Work out the finished part from the listing and answer in its coordinate system (mm). A direction names the side the tool comes from. Coordinates: 2 decimals unless noted, no trailing zeros. Loops run counter-clockwise (first coordinate to the right, second up) from the corner with the lowest first, then second, coordinate; pieces in that order, holes last. Notation, with made-up numbers: (21.25, 40.25) -> (69.25, 40.25) arc R16 cw to (69.25, 57.25) -> close; hole circle Ø3 at (-1, -10). An arc over 180 degrees is marked (long way). Use a Markdown table: item, result. Add a question column.
```python
from build123d import *

# Parameters (mm, degrees)
SKETCH8_W               = 3.38
SKETCH8_H               = 38.1
BOSS_EXTRUDE10_DEPTH    = 43.18
CUT_EXTRUDE7_DEPTH      = 71.315115907
CUT_EXTRUDE7_DEPTH_BACK = 71.315115907
SKETCH18_R              = 3.175
SKETCH23_R              = 3.175
CUT_EXTRUDE9_DEPTH      = 71.315115907


with BuildPart() as part:
    # Sketch2 → Revolve1 (revolve)
    with BuildSketch(Plane(origin=(0, 0, 0), x_dir=(1, 0, 0), z_dir=(0, 1, 0))):
        Polygon((25.408530316, 0), (25.408530316, 2.54), (26.875, 5.08), (33.225, 5.08), (33.225, 0), align=None)
    revolve(axis=Axis((0, 0, 0), (0, 0, -1)))

    # Sketch8 → Revolve2 (revolve)
    with BuildSketch(Plane(origin=(0, 0, 0), x_dir=(1, 0, 0), z_dir=(0, 1, 0)), mode=Mode.PRIVATE) as revolve2_sk:
        with Locations((-31.535, 24.13)):
            Rectangle(SKETCH8_W, SKETCH8_H)
    revolve(revolve2_sk.sketch.rotate(Axis((0, 0, 0), (0, 0, -1)), 180), axis=Axis((0, 0, 0), (0, 0, -1)))

    # Sketch19 → Boss-Extrude10 (add)
    with BuildSketch(Plane.XY):
        with BuildLine():
            Line((-6.35, 32.612545515), (-6.35, 44.45))
            Line((-6.35, 44.45), (6.35, 44.45))
            Line((6.35, 44.45), (6.35, 32.612545515))
            ThreePointArc((6.35, 32.612545515), (0, 33.225), (-6.35, 32.612545515))
        make_face()
        with BuildLine():
            Line((6.35, -44.45), (-6.35, -44.45))
            Line((-6.35, -44.45), (-6.35, -32.612545515))
            ThreePointArc((-6.35, -32.612545515), (0, -33.225), (6.35, -32.612545515))
            Line((6.35, -32.612545515), (6.35, -44.45))
        make_face()
    extrude(amount=-BOSS_EXTRUDE10_DEPTH)

    # Sketch18 → Cut-Extrude7 (cut, two sides: drawn at the far end of the back side and taken through both)
    with BuildSketch(Plane(origin=(0, 0, 0), x_dir=(0, 0, -1), z_dir=(1, 0, 0)).offset(-CUT_EXTRUDE7_DEPTH_BACK)):
        with Locations((9.525, 38.1)):
            Circle(SKETCH18_R)
        with Locations((33.655, 38.1)):
            Circle(SKETCH18_R)
        with Locations((9.525, -38.1)):
            Circle(SKETCH18_R)
        with Locations((33.655, -38.1)):
            Circle(SKETCH18_R)
    extrude(amount=CUT_EXTRUDE7_DEPTH + CUT_EXTRUDE7_DEPTH_BACK, mode=Mode.SUBTRACT)

    # Sketch23 → Cut-Extrude9 (cut, symmetric)
    with BuildSketch(Plane(origin=(0, 0, 0), x_dir=(-0.5000000000000014, 0.8660254037844378, 0), z_dir=(-0.8660254037844378, -0.5000000000000014, 0))):
        with Locations(Location((0, 21.59, 0), (0, 0, 180))):
            Circle(SKETCH23_R)
    cut_extrude9 = extrude(amount=CUT_EXTRUDE9_DEPTH, both=True, mode=Mode.SUBTRACT)

    # Mirror3: Cut-Extrude9 across plane
    add(cut_extrude9.mirror(Plane.ZX), mode=Mode.SUBTRACT)


solid = part.part
```
Item 1: Find the intervals of material crossed by probe 1 along Y at (x, z) = (0, -1); probe 2 along Y at (x, z) = (-19.5, -35); probe 3 along Z at (x, y) = (27.5, -9.5), in increasing order.
Item 2: Section A-A (x = 0) is taken. Determine the outline of the cut face in (y, z) (3 decimals).
Item 3: Section D-D (y = -38.1) is taken. Determine the outline of the cut face in (x, z), then the cut area to 3 significant figures.
Item 4: Given pin 1 (7.5 mm diameter, centred on y = -38.1, z = -9.525, fed in from -X); pin 2 (3.5 mm diameter, centred on y = 39, z = -24.5, fed in from +X); pin 3 (3 mm diameter, centred on y = 26.5, z = -38.5, fed in from +X); pin 4 (5 mm diameter, centred on y = 38.1, z = -33.655, fed in from +X), each flat-ended and moving along its own axis, determine where each tip first touches the part or whether it passes through.
Item 5: Section B-B (z = -38) is taken. Determine the outline of the cut face in (x, y) (3 decimals), then the cut area to 3 significant figures.
Item 6: For faces 4 (the face through (6.35, 39, -21)), 5 (the face through (28.47, -8.96, -24.4)), 6 (the face through (6.35, -38, -21)), 7 (the face through (-6.35, 38, -21)), determine the directions among +Z, -Z, +X, -X, +Y, -Y from which every point of the face is accessible in a straight line to the end or side of a thin tool.
Item 7: For a pull along X with two mould halves and no side action, classify faces 1 (the face through (20, -16, 0)), 2 (the face through (33.22, 0.64, -21.29)), 3 (the face through (-20.236, 15.517, -2.699)) as +X half, -X half, draft (parallel to the pull), parting line (faces both ways), or undercut.
Item 8: Section C-C (y = 0) is taken. Determine the outline of the cut face in (x, z) (3 decimals).
Output:
| question | item | result |
|---|---|---|
| 1 | probe 1 | y = -44.45 to -25.41, 25.41 to 44.45 |
| 1 | probe 2 | y = -26.9 to -22.59, 22.59 to 26.9 |
| 1 | probe 3 | z = -5.08 to 0 |
| 2 | outline | (-44.45, -43.18) -> (-29.845, -43.18) -> (-29.845, -5.08) -> (-26.875, -5.08) -> (-25.409, -2.54) -> (-25.409, 0) -> (-44.45, 0) -> close; (25.409, -2.54) -> (26.875, -5.08) -> (29.845, -5.08) -> (29.845, -43.18) -> (44.45, -43.18) -> (44.45, 0) -> (25.409, 0) -> close; hole circle Ø6.35 at (-38.1, -33.655); hole circle Ø6.35 at (-38.1, -9.525); hole circle Ø6.35 at (38.1, -33.655); hole circle Ø6.35 at (38.1, -9.525) |
| 3 | outline | (-6.35, -43.18) -> (6.35, -43.18) -> (6.35, -36.83) -> (-6.35, -36.83) -> close; (-6.35, -30.48) -> (6.35, -30.48) -> (6.35, -12.7) -> (-6.35, -12.7) -> close; (-6.35, -6.35) -> (6.35, -6.35) -> (6.35, 0) -> (-6.35, 0) -> close |
| 3 | area | 387 mm2 |
| 4 | pin 1 | stops at x = -6.35 |
| 4 | pin 2 | stops at x = 6.35 |
| 4 | pin 3 | stops at x = 21.88 |
| 4 | pin 4 | passes through |
| 5 | outline | (-6.35, -44.45) -> (6.35, -44.45) -> (6.35, -32.613) arc R33.225 ccw to (6.35, 32.613) -> (6.35, 44.45) -> (-6.35, 44.45) -> (-6.35, 32.613) arc R33.225 ccw to (-6.35, -32.613) -> close; hole circle Ø59.69 at (0, 0) |
| 5 | area | 960 mm2 |
| 6 | face 4 | +Z, -Z, +X, +Y |
| 6 | face 5 | -Z |
| 6 | face 6 | +Z, -Z, +X, -Y |
| 6 | face 7 | +Z, -Z, -X, +Y |
| 7 | face 1 | draft |
| 7 | face 2 | +X half |
| 7 | face 3 | undercut |
| 8 | outline | (-33.225, -43.18) -> (-29.845, -43.18) -> (-29.845, -5.08) -> (-26.875, -5.08) -> (-25.409, -2.54) -> (-25.409, 0) -> (-33.225, 0) -> close; (25.409, -2.54) -> (26.875, -5.08) -> (29.845, -5.08) -> (29.845, -43.18) -> (33.225, -43.18) -> (33.225, 0) -> (25.409, 0) -> close |
